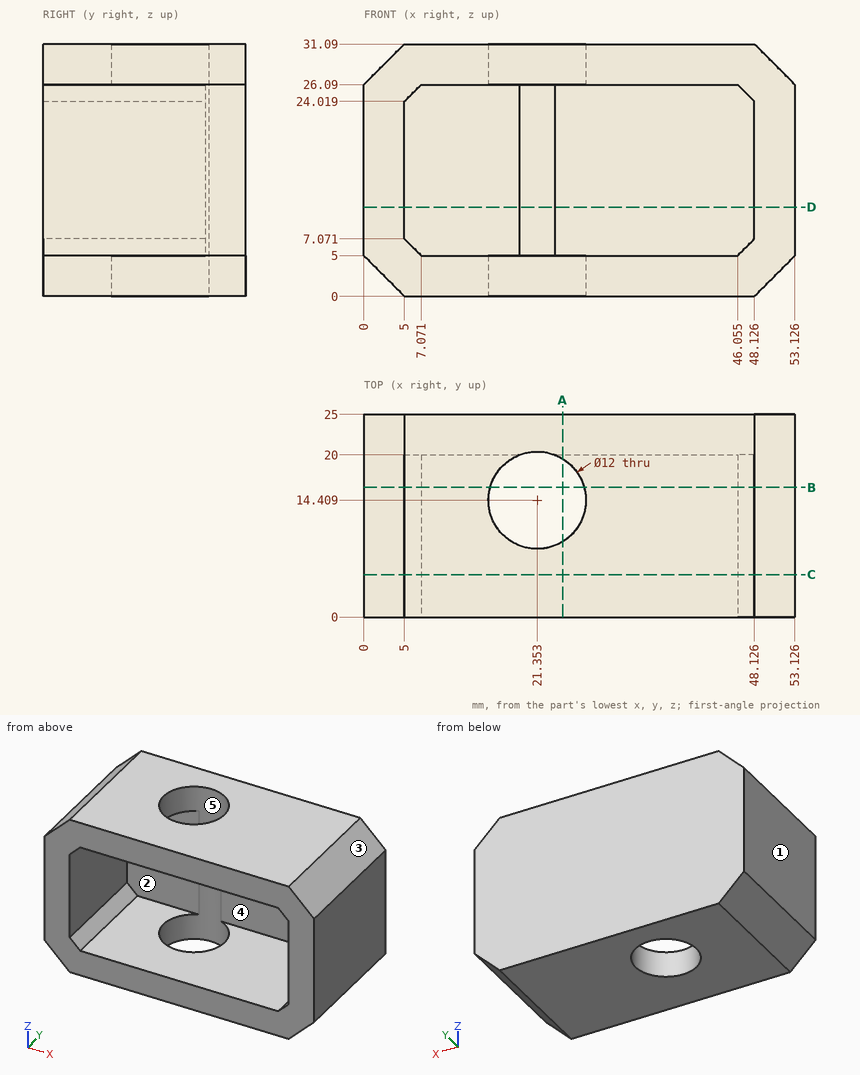
Could you check a few things on this drawing? It's one solid part, dimensions in mm from its lowest x, y, z. A direction names the side the tool comes from. Give positions to 0.01 mm unless a question says otherwise; leave off trailing zeros. Loops run counter-clockwise (first coordinate to the right, second up) from the corner with the lowest first, then second, coordinate; pieces in that order, holes last. Notation, with made-up numbers: M 82,-31 L 127,-31 A24 cw 127,-4 Z; hole C 63.5,71 d5. An arc over 180 degrees is marked long. One line per question, with ' | ' between items. Start each with the question number.
Q1. If we mould it in two halves opening along Z, with no side actions, what happens to the marked faces 1, 2 and 3? For each: +Z half, -Z half, draft (parallel to the pull), parting line (faces both ways), or undercut.
Q2. If we section it at C-C (y = 5.25): Please give me the cut outline in (x, z) (1 decimal), plus the area to 3 significant figures.
Q3. For the marked faces 4 and 5, which set-ups out of +Z, -Z, +X, -X, +Y, -Y let a thin tool reach every point of the face, with its end or its side?
Q4. If we section it at B-B (y = 16): Please give me the cut outline in (x, z) (1 decimal).
Q5. If I drill on line 1 (Z direction, x = 38, y = 14.25); line 2 (X direction, y = 6.25, z = 13); line 3 (Y direction, x = 21, z = 14), over which ranges is the centre line in solid material (lowest first)? Write a range as from..to.
Q6. If we section it at A-A (x = 24.5): Please give me the cut outline in (y, z).
Q7. For pin 1 Ø15.5 at (x, z) = (10, 14) entering from -Y; pin 2 Ø10.5 at (x, z) = (38.5, 14) entering from -Y, each with a flat end and sliding along its axis, tell me the tip position at first contact or that it passes through.
Q8. If we section it at D-D (z = 11): Please give me the cut outline in (x, y).
Computed:
1) face 1: draft | face 2: undercut | face 3: +Z half
2) outline: M 0,5 L 5,0 L 48.1,0 L 53.1,5 L 53.1,26.1 L 48.1,31.1 L 5,31.1 L 0,26.1 Z; hole M 5,7.1 L 7.1,5 L 46.1,5 L 48.1,7.1 L 48.1,24 L 46.1,26.1 L 7.1,26.1 L 5,24 Z | area: 701 mm²
3) face 4: -Y | face 5: +Z, -Z
4) outline: M 0,5 L 5,0 L 15.6,0 L 15.6,5 L 7.1,5 L 5,7.1 L 5,24 L 7.1,26.1 L 15.6,26.1 L 15.6,31.1 L 5,31.1 L 0,26.1 Z; M 27.1,0 L 48.1,0 L 53.1,5 L 53.1,26.1 L 48.1,31.1 L 27.1,31.1 L 27.1,26.1 L 46.1,26.1 L 48.1,24 L 48.1,7.1 L 46.1,5 L 27.1,5 Z
5) line 1: z = 0..5, 26.09..31.09 | line 2: x = 0..5, 48.13..53.13 | line 3: y = 20.4..25
6) outline: M 0,0 L 9.3,0 L 9.3,5 L 0,5 Z; M 0,26.09 L 9.3,26.09 L 9.3,31.09 L 0,31.09 Z; M 19.52,0 L 25,0 L 25,31.09 L 19.52,31.09 L 19.52,26.09 L 20,26.09 L 20,5 L 19.52,5 Z
7) pin 1: stops at y = 0 | pin 2: stops at y = 20
8) outline: M 0,0 L 5,0 L 5,20 L 19.18,20 A6 cw 23.53,20 L 48.13,20 L 48.13,0 L 53.13,0 L 53.13,25 L 0,25 Z
